For this review, take the finished solid that the model builds, in its own axes (mm). Face numbers are marked on the shaded views. Round coordinates to 2 decimals unless told otherwise and drop trailing zeros. Write each loop counter-clockwise with the first axis right and the second up, starting at its lowest first coordinate (ties: lowest second). Pieces come first, ordered by that corner, then holes. Notation, with made-up numbers: (-1.75, 68) - (18.25, 68) arc R12 ccw to (18.25, 89) - close; hole circle Ø7 at (-33, 55). An arc over 180 degrees is marked (long way). One line per item, written item: value. Start each with the question number.
Q1. For probe 1 along Z at (x, y) = (0, -3.75); probe 2 along Z at (x, y) = (-9, -7.25); probe 3 along Y at (x, z) = (9.5, -27), list the stretches that pass through material, from the lowest coordinate up.
Q2. Add section A-A on z = 0. Write out the cut boundary in (x, y).
Q3. Clearance check with flat-ended pins moving along their axes: pin 1 Ø1.5 at (x, z) = (21, -8) entering from -Y; pin 2 Ø23 at (x, z) = (0, 0) entering from +Y; pin 3 Ø3 at (y, z) = (-15.5, 17) entering from +X. State where each tip first meets the part, or that it passes through.
Q4. Mouldability with a two-part tool opening along Z and no side actions: class the marked faces 1, 2, 3 and 4 as +Z half, -Z half, draft (parallel to the pull), parting line (faces both ways), or undercut.
Q5. Add section D-D on y = -10.75. Write out the cut boundary in (x, z), and give its area (3 significant figures).
Q6. Add section C-C on y = -2.5. Write out the cut boundary in (x, z).
Q7. Add section B-B on x = 0. Write out the cut boundary in (y, z).
```python
from build123d import *

# Parameters (mm, degrees)
F1_DEPTH = 12.7
F2_R     = 19.05
F2_R_2   = 12.7
F3_DEPTH = 19.05
F4_R     = 5.08


with BuildPart() as f1:
    # F0 (on Front) → F1 (new body)
    with BuildSketch(Plane.XZ):
        with BuildLine():
            Line((0, 31.75), (0, 19.05))
            ThreePointArc((0, 19.05), (13.4703841816, 13.4703841816), (19.05, 0))
            ThreePointArc((19.05, 0), (-7.2901193866, -17.5999050943), (-13.4703841816, 13.4703841816))
            Line((-13.4703841816, 13.4703841816), (-31.75, 31.75))
            Line((-31.75, 31.75), (-31.75, -31.75))
            Line((-31.75, -31.75), (31.75, -31.75))
            Line((31.75, -31.75), (31.75, 31.75))
            Line((31.75, 31.75), (0, 31.75))
        make_face()
        with BuildLine():
            ThreePointArc((-13.4703841816, 13.4703841816), (-7.2901193866, 17.5999050943), (0, 19.05))
            Line((0, 19.05), (0, 31.75))
            Line((0, 31.75), (-31.75, 31.75))
            Line((-31.75, 31.75), (-13.4703841816, 13.4703841816))
        make_face()
    extrude(amount=F1_DEPTH)

    # F2 (on Front) → F3 (join)
    with BuildSketch(Plane.XZ):
        Circle(F2_R)
        Circle(F2_R_2, mode=Mode.SUBTRACT)
    extrude(amount=F3_DEPTH)

    # F4
    f4_edges = [f1.edges().sort_by_distance(p)[0] for p in [
        (-19.05, -12.7, 0),
        (0, -12.7, 31.75),
        (-31.75, -12.7, 0),
        (0, -12.7, -31.75),
        (31.75, -12.7, 0),
        (31.75, -6.35, 31.75),
        (-31.75, -6.35, 31.75),
        (-31.75, -6.35, -31.75),
        (31.75, -6.35, -31.75),
    ]]
    fillet(f4_edges, radius=F4_R)


solid = f1.part
```
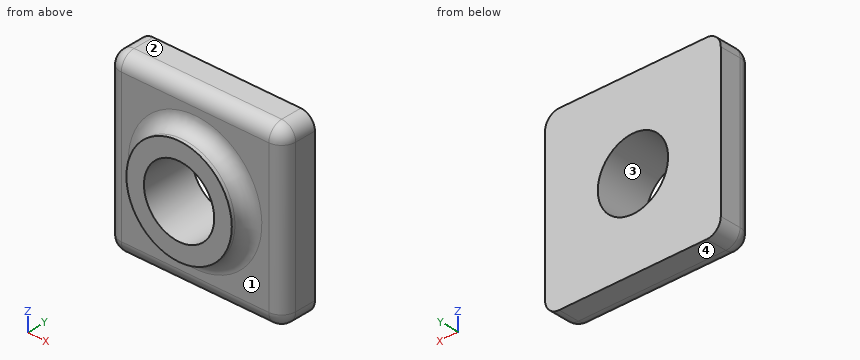
Result set:
1. probe 1: z = -31.75 to -12.7, 12.7 to 31.75
1. probe 2: z = -31.75 to -8.96, 8.96 to 31.75
1. probe 3: y = -12.69 to 0
2. outline: (-31.75, -7.62) arc R5.08 ccw to (-26.67, -12.7) - (-24.13, -12.7) arc R5.08 cw to (-19.05, -17.78) - (-19.05, -19.05) - (-12.7, -19.05) - (-12.7, 0) - (-31.75, 0) - close; (12.7, -19.05) - (19.05, -19.05) - (19.05, -17.78) arc R5.08 cw to (24.13, -12.7) - (26.67, -12.7) arc R5.08 ccw to (31.75, -7.62) - (31.75, 0) - (12.7, 0) - close
3. pin 1: stops at y = -13.31
3. pin 2: passes through
3. pin 3: stops at x = 12.58
4. face 1: draft
4. face 2: +Z half
4. face 3: undercut
4. face 4: -Z half
5. outline: (-30.67, -26.67) arc R4 ccw to (-26.67, -30.67) - (26.67, -30.67) arc R4 ccw to (30.67, -26.67) - (30.67, 26.67) arc R4 ccw to (26.67, 30.67) - (-26.67, 30.67) arc R4 ccw to (-30.67, 26.67) - close; hole circle Ø25.4 at (0, 0)
5. area: 3,240 mm^2
6. outline: (-31.75, -26.67) arc R5.08 ccw to (-26.67, -31.75) - (26.67, -31.75) arc R5.08 ccw to (31.75, -26.67) - (31.75, 26.67) arc R5.08 ccw to (26.67, 31.75) - (-26.67, 31.75) arc R5.08 ccw to (-31.75, 26.67) - close; hole circle Ø25.4 at (0, 0)
7. outline: (-19.05, -19.05) - (-17.78, -19.05) arc R5.08 cw to (-12.7, -24.13) - (-12.7, -26.67) arc R5.08 ccw to (-7.62, -31.75) - (0, -31.75) - (0, -12.7) - (-19.05, -12.7) - close; (-19.05, 12.7) - (0, 12.7) - (0, 31.75) - (-7.62, 31.75) arc R5.08 ccw to (-12.7, 26.67) - (-12.7, 24.13) arc R5.08 cw to (-17.78, 19.05) - (-19.05, 19.05) - close
